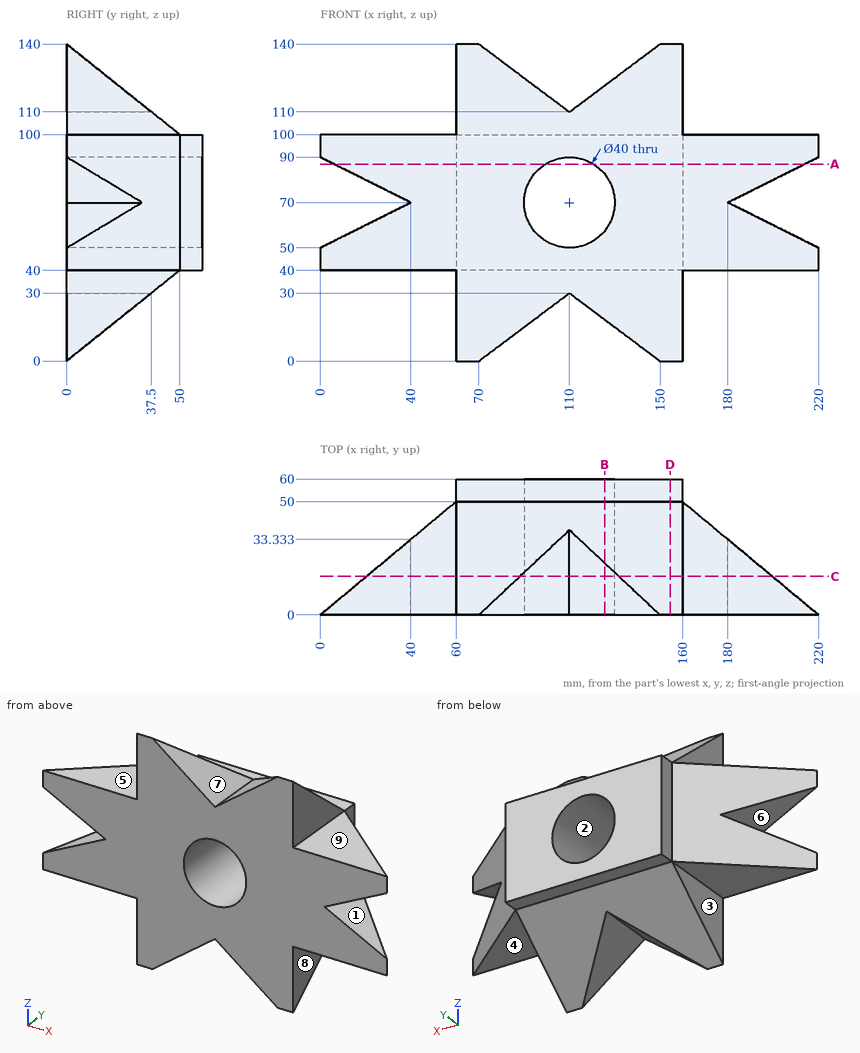
Part print with two shaded views. Sizes in mm from the minimum x, y, z corner. A direction names the side the tool comes from. Round coordinates to 2 decimals unless told otherwise and drop trailing zeros. Loops run counter-clockwise (first coordinate to the right, second up) from the corner with the lowest first, then second, coordinate; pieces in that order, holes last. Notation, with made-up numbers: (38.25, -30.5) - (76.25, -30.5) arc R18 cw to (76.25, 3.5) - close; hole circle Ø7 at (-3, 49.25). An arc over 180 degrees is marked (long way). Answer as a JSON object with one key per item and string values.
Item 1: Tool access for the marked faces 5, 6, 7, 8 and 9: list every direction of +Z, -Z, +X, -X, +Y, -Y with a clear straight run to the whole face (end or side of a thin tool).
Output:
{"face 5": "+Z, -X, +Y, -Y", "face 6": "-X, +Y, -Y", "face 7": "+Z, +Y, -Y", "face 8": "-Z, +X, +Y, -Y", "face 9": "+Z, +X, +Y, -Y"}
Item 2: Band-saw the part on A-A on z = 87. List the corners of the cut face in (x, y) (1 decimal).
Output:
{"outline": "(6, 0) - (99.5, 0) - (99.5, 60) - (60, 60) - (60, 50) - (6, 5) - close; (120.5, 0) - (214, 0) - (214, 5) - (160, 50) - (160, 60) - (120.5, 60) - close"}
Item 3: Band-saw the part on D-D on x = 154.5. List the corners of the cut face in (y, z), plus the area to 3 significant figures.
Output:
{"outline": "(0, 0) - (50, 40) - (60, 40) - (60, 100) - (50, 100) - (0, 140) - close", "area": "5,600 mm2"}
Item 4: Pull direction Z, two halves, no side cores. Call the marked faces 1, 2, 3 and 4: pulls with the +Z half, pulls with the -Z half, needs draft (parallel to the pull), parting line crosses it, or undercut.
Output:
{"face 1": "undercut", "face 2": "undercut", "face 3": "needs draft", "face 4": "pulls with the -Z half"}
Item 5: Pin check, flat tips, straight feed: pin 1 (25 mm diameter, centred on x = 192, y = 30.5, fed in from +Z); pin 2 (1.5 mm diameter, centred on x = 121, z = 118, fed in from +Y); pin 3 (20 mm diameter, centred on y = 18.5, z = 116.5, fed in from -X). Stop position of each tip, or through.
Output:
{"pin 1": "z = 100", "pin 2": "y = 28.44", "pin 3": "x = 60"}
Item 6: Band-saw the part on B-B on x = 125.5. List the corners of the cut face in (y, z) (1 decimal), plus the area to 3 significant figures.
Output:
{"outline": "(0, 18.4) - (23, 18.4) - (50, 40) - (60, 40) - (60, 57.4) - (0, 57.4) - close; (0, 82.6) - (60, 82.6) - (60, 100) - (50, 100) - (23, 121.6) - (0, 121.6) - close", "area": "3,660 mm2"}
Item 7: Wall check: L1, parallel to X at y = 29, z = 70; L2, parallel to X at y = 8, z = 88.5; L3, parallel to Z at x = 110, y = 24. Give the ranges that are in metal, low to high.
Output:
{"L1": "40 to 90, 130 to 180", "L2": "9.6 to 102.4, 117.6 to 210.4", "L3": "30 to 50, 90 to 110"}
Item 8: Band-saw the part on C-C on y = 17. List the corners of the cut face in (x, z).
Output:
{"outline": "(20.4, 40) - (60, 40) - (60, 13.6) - (88.13, 13.6) - (110, 30) - (131.87, 13.6) - (160, 13.6) - (160, 40) - (199.6, 40) - (199.6, 60.2) - (180, 70) - (199.6, 79.8) - (199.6, 100) - (160, 100) - (160, 126.4) - (131.87, 126.4) - (110, 110) - (88.13, 126.4) - (60, 126.4) - (60, 100) - (20.4, 100) - (20.4, 79.8) - (40, 70) - (20.4, 60.2) - close; hole circle Ø40 at (110, 70)"}
